Build history of the part. All positions in model axes, mm. Give positions to 0.01 mm unless a question says otherwise; leave off trailing zeros. Loops run counter-clockwise (first coordinate to the right, second up) from the corner with the lowest first, then second, coordinate; pieces in that order, holes last. Notation, with made-up numbers: (13, -13) -> (20, -13) arc R27 ccw to (20, 15) -> close; hole circle Ø1 at (81, 39.5). An arc over 180 degrees is marked (long way). Answer as a JSON object with one key per item and string values. Group by question number.
Q1. Band-saw the part on C-C, the plane z = -361. Write the cut outline in (x, y) (3 decimals).
Q2. Band-saw the part on A-A, the plane x = 1. Write the cut outline in (y, z) (3 decimals).
Q3. Drop a flat-ended pin along its axis: pin 1 (10 mm diameter, centred on x = 15, y = -2, fed in from +Z). Give the stop position or say it passes through.
Q4. Band-saw the part on B-B, the plane y = 5.5. Write the cut outline in (x, z) (3 decimals).
Q5. Wall check: probe 1 along Y at (x, z) = (3, 64.5) (3 decimals); probe 2 along X at (y, z) = (5, -202) (3 decimals). Give the ranges that are in metal, low to high. Write a range as from..to.
Autodesk Inventor part; units mm, degrees
ref_plane "YZ Plane" through (0, 0, 0) normal (1, 0, 0) x (0, 1, 0)
ref_plane "XZ Plane" through (0, 0, 0) normal (0, 1, 0) x (-1, 0, 0)
ref_plane "XY Plane" through (0, 0, 0) normal (0, 0, 1) x (1, 0, 0)
sketch "Sketch1" plane through (0, 0, 0) normal (0, 0, 1) x (1, 0, 0)
  line L0 (-35.56, 0) -> (35.56, 0)
  line L1 (0, -17.78) -> (0, 17.78)
  line L2 (-25.4, 12.7) -> (25.4, 12.7)
  line L3 (25.4, 12.7) -> (25.4, -12.7)
  line L4 (25.4, -12.7) -> (-25.4, -12.7)
  line L5 (-25.4, -12.7) -> (-25.4, 12.7)
  line L6 (22.225, 9.525) -> (-22.225, 9.525)
  line L7 (-22.225, 9.525) -> (-22.225, -9.525)
  line L8 (-22.225, -9.525) -> (22.225, -9.525)
  line L9 (22.225, -9.525) -> (22.225, 9.525)
  point P0 (0, 0)
  point P1 (-25.4, 0)
  point P2 (0, 12.7)
  dimension "d0" = 25.4
  dimension "d1" = 3.175
  dimension "d7" = 50.8
extrude "Extrusion1" add sketch "Sketch1" along normal mid plane 914.4 contours L5 L2 L1 L6 L7 L0 | L0 L7 L8 L1 L4 L5 | L1 L8 L9 L0 L3 L4 | L2 L3 L0 L9 L6 L1
properties part number "tubing_template_0.125" material "Aluminum-6061"
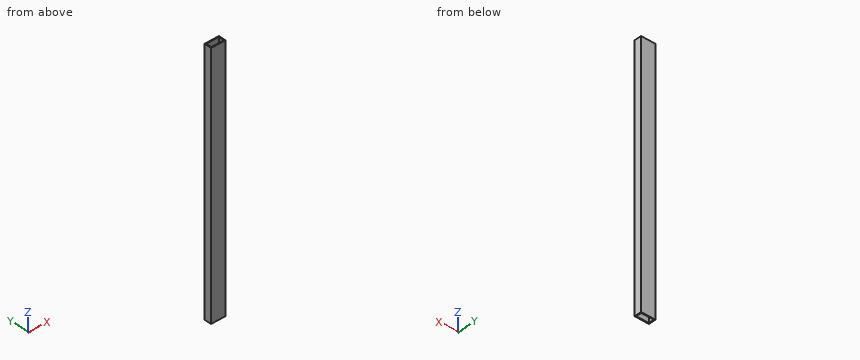
Worked answers:
{
 "1": {"outline": "(-25.4, -12.7) -> (25.4, -12.7) -> (25.4, 12.7) -> (-25.4, 12.7) -> close; hole (-22.225, -9.525) -> (22.225, -9.525) -> (22.225, 9.525) -> (-22.225, 9.525) -> close"},
 "2": {"outline": "(-12.7, -457.2) -> (-9.525, -457.2) -> (-9.525, 457.2) -> (-12.7, 457.2) -> close; (9.525, -457.2) -> (12.7, -457.2) -> (12.7, 457.2) -> (9.525, 457.2) -> close"},
 "3": {"pin 1": "through"},
 "4": {"outline": "(-25.4, -457.2) -> (-22.225, -457.2) -> (-22.225, 457.2) -> (-25.4, 457.2) -> close; (22.225, -457.2) -> (25.4, -457.2) -> (25.4, 457.2) -> (22.225, 457.2) -> close"},
 "5": {"probe 1": "-12.7..-9.525, 9.525..12.7", "probe 2": "-25.4..-22.225, 22.225..25.4"}
}
